Model file for the job. Use its own axes, mm. A direction names the side the tool comes from. Round coordinates to 2 decimals unless told otherwise and drop trailing zeros. Order: outer loops, then holes, each group sorted by start corner. A loop starts at its lowest first (then second) coordinate and runs counter-clockwise, first axis right, second up. Notation, with made-up numbers: (72.5, -6.5) - (121.5, -6.5) arc R24 ccw to (121.5, 29.5) - close; hole circle Ø3 at (88.5, -29.75). An arc over 180 degrees is marked (long way). Put each result on its own line as item: value. Start each with the question number.
Item 1: Saw through at C-C on y = 2. List the corners of the cut face in (x, z).
Item 2: Saw through at A-A on x = -19. List the corners of the cut face in (y, z).
Item 3: Probe probe 1 along Z at (x, y) = (-13, 1.85); probe 2 along X at (y, z) = (2.8, -21.5); probe 3 along X at (y, z) = (4.55, -4). List the from-to ranges inside material, lowest first.
Item 4: Saw through at B-B on z = -8.5. List the corners of the cut face in (x, y), plus the area to 3 significant figures.
Item 5: Which spindle directions (+Z, -Z, +X, -X, +Y, -Y) get a long thin tool onto all of the face, cutting with end or side? Do faces 1 (the face through (5, 2, -14)), 2 (the face through (0, 2, -14)). Say none if no direction does.
Item 6: Mould opens along Z. For faces 3 (the face through (-23, 5, 3)), 4 (the face through (-23, 2, 5)), 5 (the face through (-2.789, 2.465, -25.132)), 6 (the face through (-46, 2, -14)) say: pulls with the +Z half, pulls with the -Z half, needs draft (parallel to the pull), parting line crosses it, or undercut.
Autodesk Inventor part; units mm, degrees
ref_plane "YZ Plane" through (0, 0, 0) normal (1, 0, 0) x (0, 1, 0)
ref_plane "XZ Plane" through (0, 0, 0) normal (0, 1, 0) x (-1, 0, 0)
ref_plane "XY Plane" through (0, 0, 0) normal (0, 0, 1) x (1, 0, 0)
sketch "Sketch1" plane through (0, 0, 0) normal (0, 1, 0) x (-1, 0, 0)
  line L0 (5.6569, 0) -> (36, 0)
  line L1 (36, 0) -> (36, -28)
  line L2 (36, -28) -> (5.6569, -28)
  line L3 (0, -28) -> (0, -5.6568)
  line L4 (0, 0) -> (0, -5.6568)
  line L5 (0, -5.6568) -> (5.6569, 0)
  line L6 (36, -14) -> (0, -14) construction
  line L7 (5.6569, -28) -> (36, -28)
  line L8 (0, 0) -> (0, -22.3432)
  line L9 (0, -22.3432) -> (5.6569, -28)
  line L10 (41, -28) -> (41, 5) construction
  line L11 (41, 5) -> (3.5859, 5) construction
  line L12 (3.5859, 5) -> (-3.5355, -2.1212) construction
  line L13 (36, -33) -> (5.6569, -33) construction
  line L14 (36, 0) -> (46, 0) construction
  line L15 (46, 0) -> (46, -28) construction
  line L16 (46, -28) -> (36, -28) construction
  line L17 (36, -28) -> (36, 0) construction
  line L18 (51, 5) -> (31, 5) construction
  line L19 (31, 5) -> (31, -33) construction
  line L20 (31, -33) -> (51, -33) construction
  line L21 (51, -33) -> (51, 5) construction
  line L22 (0, 0) -> (-5, 0) construction
  line L23 (-5, 0) -> (-5, -8.8109) construction
  line L24 (-5, -8.8109) -> (0, -8.8109) construction
  line L25 (0, -8.8109) -> (0, 0) construction
  line L26 (51, 5) -> (-5, 5)
  line L27 (-5, 5) -> (-5, -33.0002)
  line L28 (-5, -33.0002) -> (51, -33.0002)
  line L29 (51, -33.0002) -> (51, 5)
  line L30 (36, 0) -> (46, 0)
  line L31 (46, 0) -> (46, -28)
  line L32 (46, -28) -> (36, -28)
  line L33 (36, -28) -> (36, 0)
  dimension "d0" = 36
  dimension "d1" = 28
  dimension "d3" = 8
  dimension "d4" = 5
  dimension "d5" = 5
  dimension "d6" = 10
  dimension "d7" = 5
  dimension "d8" = 5
extrude "Extrusion1" add sketch "Sketch1" along normal blind 5
properties part number "power_test"
Results found:
1. outline: (-51, -33) - (5, -33) - (5, 5) - (-51, 5) - close; hole (-46, -28) - (-5.66, -28) - (0, -22.34) - (0, -5.66) - (-5.66, 0) - (-46, 0) - close
2. outline: (0, -33) - (5, -33) - (5, -28) - (0, -28) - close; (0, 0) - (5, 0) - (5, 5) - (0, 5) - close
3. probe 1: z = -33 to -28, 0 to 5
3. probe 2: x = -51 to -46, 0 to 5
3. probe 3: x = -51 to -46, -1.66 to 5
4. outline: (-51, 0) - (-46, 0) - (-46, 5) - (-51, 5) - close; (0, 0) - (5, 0) - (5, 5) - (0, 5) - close
4. area: 50.0 mm²
5. face 1: +Z, -Z, +X, +Y, -Y
5. face 2: +Y, -Y
6. face 3: needs draft
6. face 4: pulls with the +Z half
6. face 5: undercut
6. face 6: undercut
